Check sheet for the drawn part. Datum: minimum x, y, z corner. Units: mm. A direction names the side the tool comes from. Coordinates: 2 decimals unless noted, no trailing zeros. Loops run counter-clockwise (first coordinate to the right, second up) from the corner with the lowest first, then second, coordinate; pieces in that order, holes last.
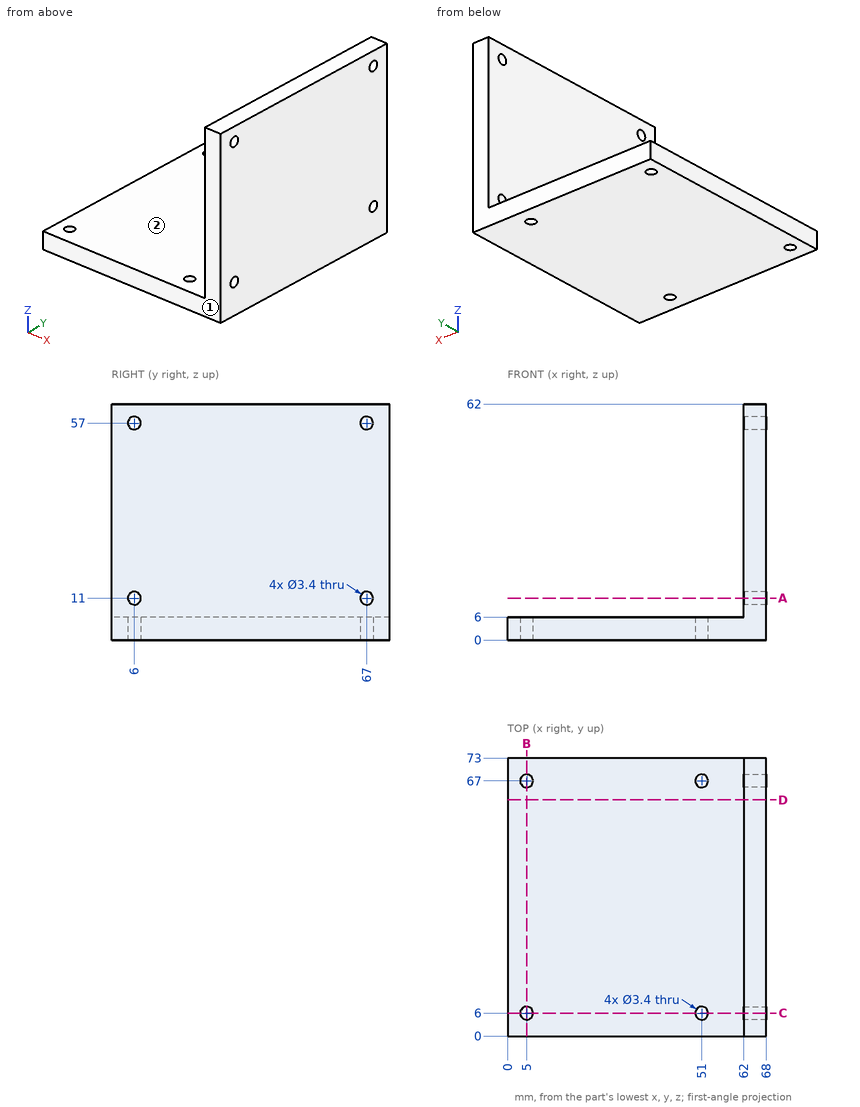
1) Section check C-C on y = 6. Enter the section's corners in (x, z), plus the area to 3 significant figures.
Answer sheet:
outline: (0, 0) - (3.3, 0) - (3.3, 6) - (0, 6) - close; (6.7, 0) - (49.3, 0) - (49.3, 6) - (6.7, 6) - close; (52.7, 0) - (68, 0) - (68, 9.3) - (62, 9.3) - (62, 6) - (52.7, 6) - close; (62, 12.7) - (68, 12.7) - (68, 55.3) - (62, 55.3) - close; (62, 58.7) - (68, 58.7) - (68, 62) - (62, 62) - close
area: 662 mm2
2) Section check B-B on x = 5. Enter the section's corners in (y, z), plus the area to 3 significant figures.
Answer sheet:
outline: (0, 0) - (4.3, 0) - (4.3, 6) - (0, 6) - close; (7.7, 0) - (65.3, 0) - (65.3, 6) - (7.7, 6) - close; (68.7, 0) - (73, 0) - (73, 6) - (68.7, 6) - close
area: 397 mm2
3) Scan lines: line 1 (Z direction, x = 65.05, y = 67); line 2 (Y direction, x = 51, z = 3.95); line 3 (X direction, y = 13, z = 17). Record each from-to range of solid material in increasing order.
Answer sheet:
line 1: z = 0 to 9.3, 12.7 to 55.3, 58.7 to 62
line 2: y = 0 to 4.3, 7.7 to 65.3, 68.7 to 73
line 3: x = 62 to 68
4) Section check D-D on y = 62. Enter the section's corners in (x, z).
Answer sheet:
outline: (0, 0) - (68, 0) - (68, 62) - (62, 62) - (62, 6) - (0, 6) - close
5) Depth check by flat-ended pin: pin 1 (1.5 mm diameter, centred on x = 25, y = 11.5, fed in from +Z); pin 2 (4 mm diameter, centred on y = 6, z = 57, fed in from +X); pin 3 (5.5 mm diameter, centred on y = 67, z = 11, fed in from -X). Enter the tip coordinate at first touch or a pass-through.
Answer sheet:
pin 1: stops at z = 6
pin 2: stops at x = 68
pin 3: stops at x = 62
6) Set-up check for the marked faces 1 and 2: record each of +Z, -Z, +X, -X, +Y, -Y from which the full face is reachable in a straight line by a thin tool's end or side.
Answer sheet:
face 1: +Z, -Z, +X, -X, -Y
face 2: +Z, -X, +Y, -Y
7) Section check A-A on z = 11. Enter the section's corners in (x, y).
Answer sheet:
outline: (62, 0) - (68, 0) - (68, 4.3) - (62, 4.3) - close; (62, 7.7) - (68, 7.7) - (68, 65.3) - (62, 65.3) - close; (62, 68.7) - (68, 68.7) - (68, 73) - (62, 73) - close
